```python
from build123d import *

# Parameters (mm, degrees)
BOSS_EXTRUDE1_DEPTH = 609.6
SKETCH3_W           = 635.2
SKETCH3_H           = 25.4
CUT_EXTRUDE2_DEPTH  = 30.48
SKETCH5_R           = 1.7
CUT_EXTRUDE3_DEPTH  = 611.137198198
SKETCH7_R           = 1.7
CUT_EXTRUDE4_DEPTH  = 611.137198198


with BuildPart() as part:
    # Sketch2 → Boss-Extrude1 (new, symmetric)
    with BuildSketch(Plane.XY):
        with BuildLine():
            Line((-12.7, -12.7), (12.7, -12.7))
            Line((12.7, -12.7), (12.7, 12.7))
            Line((12.7, 12.7), (11.1125, 12.7))
            ThreePointArc((11.1125, 12.7), (9.989967985, 12.235032015), (9.525, 11.1125))
            Line((9.525, 11.1125), (9.525, -6.35))
            ThreePointArc((9.525, -6.35), (8.59506403, -8.59506403), (6.35, -9.525))
            Line((6.35, -9.525), (-11.1125, -9.525))
            ThreePointArc((-11.1125, -9.525), (-12.235032015, -9.989967985), (-12.7, -11.1125))
            Line((-12.7, -11.1125), (-12.7, -12.7))
        make_face()
    extrude(amount=BOSS_EXTRUDE1_DEPTH, both=True)

    # Sketch3 → Cut-Extrude2 (cut)
    with BuildSketch(Plane(origin=(12.7, 0, 0), x_dir=(0, 0, -1), z_dir=(1, 0, 0))):
        with Locations((292, 0)):
            Rectangle(SKETCH3_W, SKETCH3_H)
    extrude(amount=-CUT_EXTRUDE2_DEPTH, mode=Mode.SUBTRACT)

    # Sketch5 → Cut-Extrude3 (cut, through all)
    with BuildSketch(Plane.ZY.offset(-9.525)):
        with Locations(Location((78.35, 2.38125, 0), (0, 0, 270))):
            Circle(SKETCH5_R)
        with Locations(Location((92.85, 2.38125, 0), (0, 0, 270))):
            Circle(SKETCH5_R)
        with Locations(Location((107.35, 2.38125, 0), (0, 0, 270))):
            Circle(SKETCH5_R)
        with Locations(Location((121.85, 2.38125, 0), (0, 0, 270))):
            Circle(SKETCH5_R)
        with Locations(Location((136.35, 2.38125, 0), (0, 0, 270))):
            Circle(SKETCH5_R)
        with Locations(Location((150.85, 2.38125, 0), (0, 0, 270))):
            Circle(SKETCH5_R)
        with Locations(Location((165.35, 2.38125, 0), (0, 0, 270))):
            Circle(SKETCH5_R)
        with Locations(Location((179.85, 2.38125, 0), (0, 0, 270))):
            Circle(SKETCH5_R)
        with Locations(Location((194.35, 2.38125, 0), (0, 0, 270))):
            Circle(SKETCH5_R)
        with Locations(Location((208.85, 2.38125, 0), (0, 0, 270))):
            Circle(SKETCH5_R)
        with Locations(Location((223.35, 2.38125, 0), (0, 0, 270))):
            Circle(SKETCH5_R)
        with Locations(Location((237.85, 2.38125, 0), (0, 0, 270))):
            Circle(SKETCH5_R)
        with Locations(Location((252.35, 2.38125, 0), (0, 0, 270))):
            Circle(SKETCH5_R)
        with Locations(Location((266.85, 2.38125, 0), (0, 0, 270))):
            Circle(SKETCH5_R)
        with Locations(Location((281.35, 2.38125, 0), (0, 0, 270))):
            Circle(SKETCH5_R)
        with Locations(Location((295.85, 2.38125, 0), (0, 0, 270))):
            Circle(SKETCH5_R)
        with Locations(Location((310.35, 2.38125, 0), (0, 0, 270))):
            Circle(SKETCH5_R)
        with Locations(Location((324.85, 2.38125, 0), (0, 0, 270))):
            Circle(SKETCH5_R)
        with Locations(Location((339.35, 2.38125, 0), (0, 0, 270))):
            Circle(SKETCH5_R)
        with Locations(Location((353.85, 2.38125, 0), (0, 0, 270))):
            Circle(SKETCH5_R)
        with Locations(Location((368.35, 2.38125, 0), (0, 0, 270))):
            Circle(SKETCH5_R)
        with Locations(Location((382.85, 2.38125, 0), (0, 0, 270))):
            Circle(SKETCH5_R)
        with Locations(Location((397.35, 2.38125, 0), (0, 0, 270))):
            Circle(SKETCH5_R)
        with Locations(Location((411.85, 2.38125, 0), (0, 0, 270))):
            Circle(SKETCH5_R)
        with Locations(Location((426.35, 2.38125, 0), (0, 0, 270))):
            Circle(SKETCH5_R)
        with Locations(Location((440.85, 2.38125, 0), (0, 0, 270))):
            Circle(SKETCH5_R)
        with Locations(Location((455.35, 2.38125, 0), (0, 0, 270))):
            Circle(SKETCH5_R)
        with Locations(Location((469.85, 2.38125, 0), (0, 0, 270))):
            Circle(SKETCH5_R)
        with Locations(Location((484.35, 2.38125, 0), (0, 0, 270))):
            Circle(SKETCH5_R)
        with Locations(Location((498.85, 2.38125, 0), (0, 0, 270))):
            Circle(SKETCH5_R)
        with Locations(Location((513.35, 2.38125, 0), (0, 0, 270))):
            Circle(SKETCH5_R)
        with Locations(Location((527.85, 2.38125, 0), (0, 0, 270))):
            Circle(SKETCH5_R)
        with Locations(Location((542.35, 2.38125, 0), (0, 0, 270))):
            Circle(SKETCH5_R)
        with Locations(Location((556.85, 2.38125, 0), (0, 0, 270))):
            Circle(SKETCH5_R)
    extrude(amount=-CUT_EXTRUDE3_DEPTH, mode=Mode.SUBTRACT)

    # Sketch7 → Cut-Extrude4 (cut, through all)
    with BuildSketch(Plane(origin=(0, -9.525, 0), x_dir=(1, 0, 0), z_dir=(0, 1, 0))):
        with Locations(Location((-2.38125, -78.35, 0), (0, 0, 180))):
            Circle(SKETCH7_R)
        with Locations(Location((-2.38125, -92.85, 0), (0, 0, 180))):
            Circle(SKETCH7_R)
        with Locations(Location((-2.38125, -107.35, 0), (0, 0, 180))):
            Circle(SKETCH7_R)
        with Locations(Location((-2.38125, -121.85, 0), (0, 0, 180))):
            Circle(SKETCH7_R)
        with Locations(Location((-2.38125, -136.35, 0), (0, 0, 180))):
            Circle(SKETCH7_R)
        with Locations(Location((-2.38125, -150.85, 0), (0, 0, 180))):
            Circle(SKETCH7_R)
        with Locations(Location((-2.38125, -165.35, 0), (0, 0, 180))):
            Circle(SKETCH7_R)
        with Locations(Location((-2.38125, -179.85, 0), (0, 0, 180))):
            Circle(SKETCH7_R)
        with Locations(Location((-2.38125, -194.35, 0), (0, 0, 180))):
            Circle(SKETCH7_R)
        with Locations(Location((-2.38125, -208.85, 0), (0, 0, 180))):
            Circle(SKETCH7_R)
        with Locations(Location((-2.38125, -223.35, 0), (0, 0, 180))):
            Circle(SKETCH7_R)
        with Locations(Location((-2.38125, -237.85, 0), (0, 0, 180))):
            Circle(SKETCH7_R)
        with Locations(Location((-2.38125, -252.35, 0), (0, 0, 180))):
            Circle(SKETCH7_R)
        with Locations(Location((-2.38125, -266.85, 0), (0, 0, 180))):
            Circle(SKETCH7_R)
        with Locations(Location((-2.38125, -281.35, 0), (0, 0, 180))):
            Circle(SKETCH7_R)
        with Locations(Location((-2.38125, -295.85, 0), (0, 0, 180))):
            Circle(SKETCH7_R)
        with Locations(Location((-2.38125, -310.35, 0), (0, 0, 180))):
            Circle(SKETCH7_R)
        with Locations(Location((-2.38125, -324.85, 0), (0, 0, 180))):
            Circle(SKETCH7_R)
        with Locations(Location((-2.38125, -339.35, 0), (0, 0, 180))):
            Circle(SKETCH7_R)
        with Locations(Location((-2.38125, -353.85, 0), (0, 0, 180))):
            Circle(SKETCH7_R)
        with Locations(Location((-2.38125, -368.35, 0), (0, 0, 180))):
            Circle(SKETCH7_R)
        with Locations(Location((-2.38125, -382.85, 0), (0, 0, 180))):
            Circle(SKETCH7_R)
        with Locations(Location((-2.38125, -397.35, 0), (0, 0, 180))):
            Circle(SKETCH7_R)
        with Locations(Location((-2.38125, -411.85, 0), (0, 0, 180))):
            Circle(SKETCH7_R)
        with Locations(Location((-2.38125, -426.35, 0), (0, 0, 180))):
            Circle(SKETCH7_R)
        with Locations(Location((-2.38125, -440.85, 0), (0, 0, 180))):
            Circle(SKETCH7_R)
        with Locations(Location((-2.38125, -455.35, 0), (0, 0, 180))):
            Circle(SKETCH7_R)
        with Locations(Location((-2.38125, -469.85, 0), (0, 0, 180))):
            Circle(SKETCH7_R)
        with Locations(Location((-2.38125, -484.35, 0), (0, 0, 180))):
            Circle(SKETCH7_R)
        with Locations(Location((-2.38125, -498.85, 0), (0, 0, 180))):
            Circle(SKETCH7_R)
        with Locations(Location((-2.38125, -513.35, 0), (0, 0, 180))):
            Circle(SKETCH7_R)
        with Locations(Location((-2.38125, -527.85, 0), (0, 0, 180))):
            Circle(SKETCH7_R)
        with Locations(Location((-2.38125, -542.35, 0), (0, 0, 180))):
            Circle(SKETCH7_R)
        with Locations(Location((-2.38125, -556.85, 0), (0, 0, 180))):
            Circle(SKETCH7_R)
    extrude(amount=-CUT_EXTRUDE4_DEPTH, mode=Mode.SUBTRACT)


solid = part.part
```
The model under review builds one solid part; all positions refer to its coordinate system, in mm. A direction names the side the tool comes from. Round coordinates to 2 decimals unless told otherwise and drop trailing zeros.
1) Clearance check with flat-ended pins moving along their axes: P1, Ø4.5, axis at x = -2.38, z = 440.85, coming from the +Y side (3 decimals); P2, Ø2, axis at y = -7.5, z = 290, coming from the -X side; P3, Ø1, axis at y = 9, z = 214, coming from the -X side (3 decimals). State where each tip first meets the part, or that it passes through.
Values follow:
P1: stops at y = -9.525
P2: stops at x = 8.69
P3: stops at x = 9.525
2) Wall thickness on line 1 along X through (y, z) = (-11.6, 368.35); line 2 along Y through (x, z) = (11.15, 324.85); line 3 along X through (y, z) = (4.75, 380) (3 decimals): over which ranges is each line inside the solid? List them lowest first.
Values follow:
line 1: x = -12.7 to -4.08, -0.68 to 12.7
line 2: y = -12.7 to 0.68, 4.08 to 12.7
line 3: x = 9.525 to 12.7
3) Tool access review of faces 1 (the face through (7.6, -9.5, 25.6)), 2 (the face through (9.525, 3, 322)): name each direction out of +Z, -Z, +X, -X, +Y, -Y from which nothing blocks a thin tool from reaching the whole face with its end or side.
Values follow:
face 1: -Z, +X, -X, +Y, -Y
face 2: +Z, -Z, -X, +Y
